```python
from build123d import *

# Parameters (mm, degrees)
F0_R     = 175
F1_DEPTH = 31.75


with BuildPart() as f1:
    # F0 (on Top) → F1 (new body)
    with BuildSketch(Plane.XY):
        Circle(F0_R)
        with BuildLine():
            ThreePointArc((0, -129), (-6.010408, -126.510408), (-8.5, -120.5))
            Line((-8.5, -120.5), (-8.5, -32.5))
            ThreePointArc((-8.5, -32.5), (-6.010408, -26.489592), (0, -24))
            ThreePointArc((0, -24), (6.010408, -26.489592), (8.5, -32.5))
            Line((8.5, -32.5), (8.5, -120.5))
            ThreePointArc((8.5, -120.5), (6.010408, -126.510408), (0, -129))
        make_face(mode=Mode.SUBTRACT)
        with BuildLine():
            ThreePointArc((-129, 0), (-126.510408, 6.010408), (-120.5, 8.5))
            Line((-120.5, 8.5), (-32.5, 8.5))
            ThreePointArc((-32.5, 8.5), (-26.489592, 6.010408), (-24, 0))
            ThreePointArc((-24, 0), (-26.489592, -6.010408), (-32.5, -8.5))
            Line((-32.5, -8.5), (-120.5, -8.5))
            ThreePointArc((-120.5, -8.5), (-126.510408, -6.010408), (-129, 0))
        make_face(mode=Mode.SUBTRACT)
        with BuildLine():
            ThreePointArc((129, 0), (126.510408, -6.010408), (120.5, -8.5))
            Line((120.5, -8.5), (32.5, -8.5))
            ThreePointArc((32.5, -8.5), (26.489592, -6.010408), (24, 0))
            ThreePointArc((24, 0), (26.489592, 6.010408), (32.5, 8.5))
            Line((32.5, 8.5), (120.5, 8.5))
            ThreePointArc((120.5, 8.5), (126.510408, 6.010408), (129, 0))
        make_face(mode=Mode.SUBTRACT)
        with BuildLine():
            Line((-8.5, 32.5), (-8.5, 120.5))
            ThreePointArc((-8.5, 120.5), (-6.010408, 126.510408), (0, 129))
            ThreePointArc((0, 129), (6.010408, 126.510408), (8.5, 120.5))
            Line((8.5, 120.5), (8.5, 32.5))
            ThreePointArc((8.5, 32.5), (6.010408, 26.489592), (0, 24))
            ThreePointArc((0, 24), (-6.010408, 26.489592), (-8.5, 32.5))
        make_face(mode=Mode.SUBTRACT)
    extrude(amount=F1_DEPTH)


solid = f1.part
```
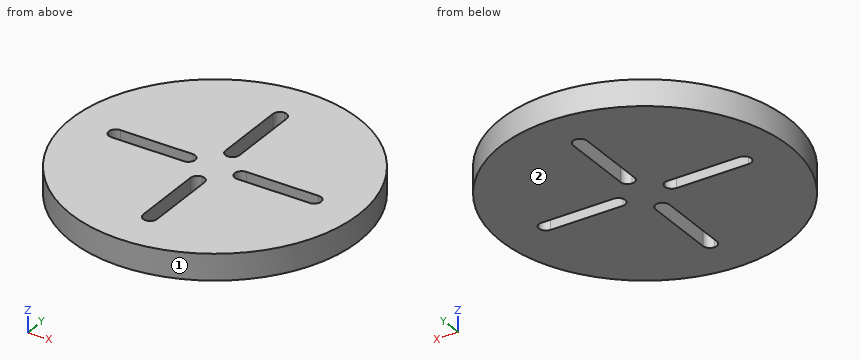
Here's how the part is built. I have some questions about the finished solid (model axes, mm). Face numbers are marked on the shaded views. Give positions to 0.01 mm unless a question says otherwise; leave off trailing zeros. Loops run counter-clockwise (first coordinate to the right, second up) from the corner with the lowest first, then second, coordinate; pieces in that order, holes last. Notation, with made-up numbers: M 89,-23.75 L 117,-23.75 A10 ccw 117,-14.75 Z; hole C 57,-6 d1. An arc over 180 degrees is marked long. Use one line per item in the form item = value. Start each with the question number.
Q1. If we section it at C-C (z = 16): Write out the boundary of the cut face in (x, y).
Q2. I need wall thicknesses on line 1 along X through (y, z) = (6, 25); line 2 along Y through (x, z) = (42.5, 5.5); line 3 along X through (y, z) = (-53, 16.5). Which ranges of each line are inside material? Lowest first, please.
Q3. If we section it at D-D (y = 143): Write out the boundary of the cut face in (x, z).
Q4. If we section it at B-B (y = 60.5): Write out the boundary of the cut face in (x, z).
Q5. If we section it at A-A (x = 64.5): Write out the boundary of the cut face in (y, z).
Q6. Thinking about a two-plate mould opening in Y: for the marked faces 1 and 2, which applies, +Y half, -Y half, draft (parallel to the pull), parting line (faces both ways), or undercut?
Q7. Will these pins go through, and if not, where does the flat tip stop? pin 1 Ø9.5 at (x, z) = (84, 14.5) entering from +Y; pin 2 Ø9.5 at (y, z) = (-89.5, 14.5) entering from -X; pin 3 Ø12 at (y, z) = (-15.5, 26.5) entering from -X.
Taken from the geometry:
q1.outline = C 0,0 d350; hole M -129,0 A8.5 ccw -120.5,-8.5 L -32.5,-8.5 A8.5 ccw -24,0 A8.5 ccw -32.5,8.5 L -120.5,8.5 A8.5 ccw Z; hole M -8.5,-120.5 A8.5 ccw 0,-129 A8.5 ccw 8.5,-120.5 L 8.5,-32.5 A8.5 ccw 0,-24 A8.5 ccw -8.5,-32.5 Z; hole M -8.5,32.5 A8.5 ccw 0,24 A8.5 ccw 8.5,32.5 L 8.5,120.5 A8.5 ccw 0,129 A8.5 ccw -8.5,120.5 Z; hole M 24,0 A8.5 ccw 32.5,-8.5 L 120.5,-8.5 A8.5 ccw 129,0 A8.5 ccw 120.5,8.5 L 32.5,8.5 A8.5 ccw Z
q2.line_1 = -174.9 to -126.52, -26.48 to 26.48, 126.52 to 174.9
q2.line_2 = -169.76 to -8.5, 8.5 to 169.76
q2.line_3 = -166.78 to -8.5, 8.5 to 166.78
q3.outline = M -100.88,0 L 100.88,0 L 100.88,31.75 L -100.88,31.75 Z
q4.outline = M -164.21,0 L -8.5,0 L -8.5,31.75 L -164.21,31.75 Z; M 8.5,0 L 164.21,0 L 164.21,31.75 L 8.5,31.75 Z
q5.outline = M -162.68,0 L -8.5,0 L -8.5,31.75 L -162.68,31.75 Z; M 8.5,0 L 162.68,0 L 162.68,31.75 L 8.5,31.75 Z
q6.face_1 = parting line
q6.face_2 = draft
q7.pin_1 = 156.03
q7.pin_2 = -153.11
q7.pin_3 = -174.74
